Input: part model. Units: mm. Frame: model coordinates. A direction names the side the tool comes from. Give positions to 0.01 mm unless a question says otherwise; leave off trailing zeros. Write each loop counter-clockwise with the first axis right and the second up, starting at its lowest first coordinate (ties: lowest second). Pieces come first, ordered by that corner, then holes. Notation, with made-up numbers: (-36, 52.25) -> (-23, 52.25) arc R35 ccw to (-23, 88.25) -> close; hole circle Ø7 at (40.5, 34.25). An arc over 180 degrees is marked (long way). Answer as a JSON object with one key per item and string values. Group by question number.
Solid Edge part; units mm, degrees
sketch "Sketch1" plane through (0, 0, 0) normal (0, -1, 0) x (1, 0, 0)
  line L0 (-42.5, 29.95) -> (-42.5, -29.95)
  line L1 (72.5, -29.95) -> (-42.5, -29.95)
  line L2 (72.5, -29.95) -> (72.5, -20.05)
  line L3 (42.5, -20.05) -> (72.5, -20.05)
  line L4 (42.5, 19.95) -> (42.5, -20.05)
  line L5 (72.5, 19.95) -> (42.5, 19.95)
  line L6 (72.5, 29.95) -> (72.5, 19.95)
  line L7 (-42.5, 29.95) -> (72.5, 29.95)
  dimension "D1" = 42.5
extrude "Protrusion1" add sketch "Sketch1" along normal mid plane 15
sketch "Sketch2" plane through (0, -7.5, 0) normal (0, -1, 0) x (1, 0, 0)
  circle A0 centre (-7.5, 0) radius 9.75
extrude "Ausschnitt_1" cut sketch "Sketch2" against normal blind 113.5793
1. Reachability of faces 1 (the face through (3, -7.5, 0)), 2 (the face through (57, 0, -20.05)) from +Z, -Z, +X, -X, +Y, -Y: full face, straight path, thin tool, end or side. Return the list, or none.
2. Section D-D (z = -12). Return the cut outline in (x, y).
3. Section A-A (x = 53.5). Return the cut outline in (y, z).
4. Contact query for flat-ended pins moving along their axis: pin 1 Ø3 at (y, z) = (4.5, -5) entering from +X; pin 2 Ø6 at (x, z) = (-15, 5) entering from +Y. Output: stop coordinate, or through.
5. Mould query, pull axis Z, two halves, no side actions, for faces 3 (the face through (1.8, -0.11, 2.93)), 4 (the face through (72.5, 0, 25)), 5 (the face through (58, 0, 19.95)), 6 (the face through (16, 0, -29.95)). Classes: pulls with the +Z half, pulls with the -Z half, needs draft (parallel to the pull), parting line crosses it, or undercut.
6. Line query: line 1 (Z direction, x = -7.5, y = 4); line 2 (Z direction, x = 66, y = -1.25); line 3 (X direction, y = -7, z = 12.5). Output: solid intervals per line, ascending.
7. Section C-C (y = -5). Return the cut outline in (x, z), plus the area to 3 significant figures.
8. Section B-B (z = 0). Return the cut outline in (x, y).
Working result:
{
 "1": {"face 1": "+Z, -Z, +X, -X, -Y", "face 2": "+X, +Y, -Y"},
 "2": {"outline": "(-42.5, -7.5) -> (42.5, -7.5) -> (42.5, 7.5) -> (-42.5, 7.5) -> close"},
 "3": {"outline": "(-7.5, -29.95) -> (7.5, -29.95) -> (7.5, -20.05) -> (-7.5, -20.05) -> close; (-7.5, 19.95) -> (7.5, 19.95) -> (7.5, 29.95) -> (-7.5, 29.95) -> close"},
 "4": {"pin 1": "stops at x = 42.5", "pin 2": "stops at y = 7.5"},
 "5": {"face 3": "undercut", "face 4": "needs draft", "face 5": "undercut", "face 6": "pulls with the -Z half"},
 "6": {"line 1": "z = -29.95 to -9.75, 9.75 to 29.95", "line 2": "z = -29.95 to -20.05, 19.95 to 29.95", "line 3": "x = -42.5 to 42.5"},
 "7": {"outline": "(-42.5, -29.95) -> (72.5, -29.95) -> (72.5, -20.05) -> (42.5, -20.05) -> (42.5, 19.95) -> (72.5, 19.95) -> (72.5, 29.95) -> (-42.5, 29.95) -> close; hole circle Ø19.5 at (-7.5, 0)", "area": "5,390 mm^2"},
 "8": {"outline": "(-42.5, -7.5) -> (-17.25, -7.5) -> (-17.25, 7.5) -> (-42.5, 7.5) -> close; (2.25, -7.5) -> (42.5, -7.5) -> (42.5, 7.5) -> (2.25, 7.5) -> close"}
}
